Print and shaded views of the part. All mm, measured from the part's lowest x, y and z. A direction names the side the tool comes from. Give positions to 0.01 mm unless a question says otherwise; leave off trailing zeros. Loops run counter-clockwise (first coordinate to the right, second up) from the corner with the lowest first, then second, coordinate; pieces in that order, holes last. Notation, with made-up numbers: (56.5, 18) - (88.5, 18) arc R36 ccw to (88.5, 55) - close; hole circle Ø10 at (46.5, 87). An arc over 180 degrees is marked (long way). Return JSON: item names as keys, results as strings.
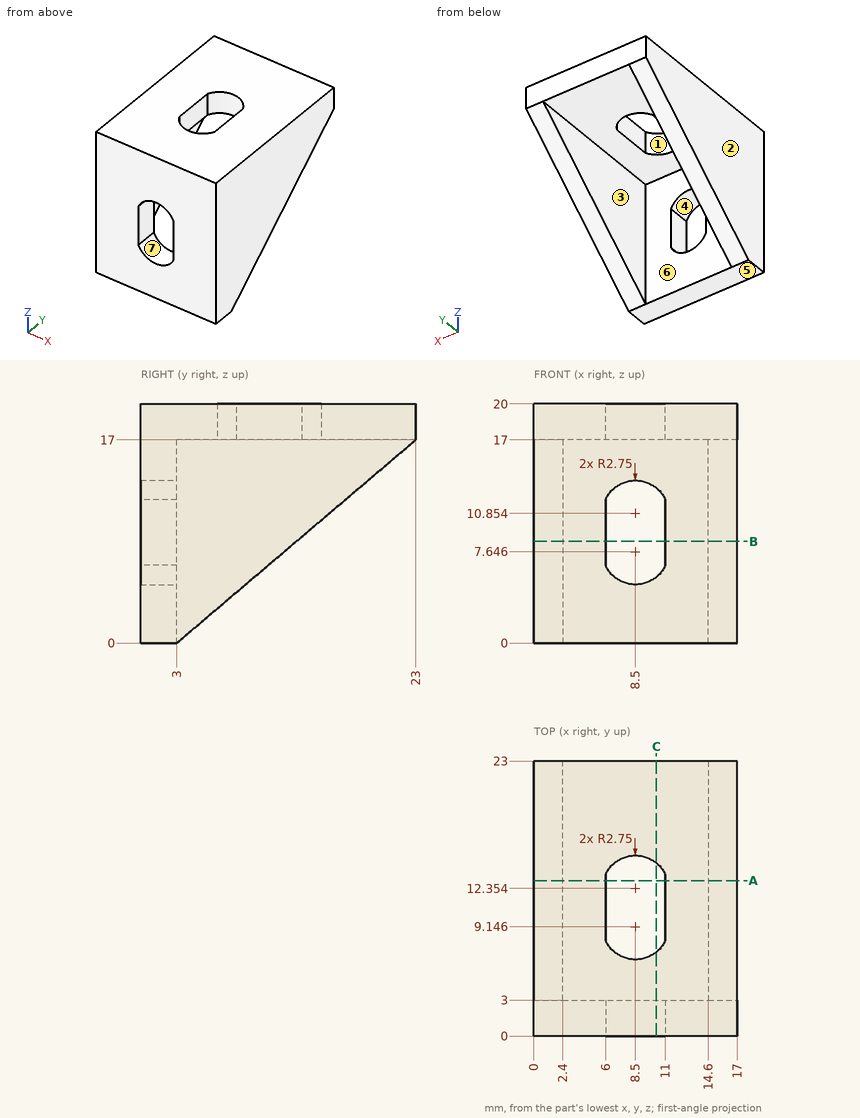
1. Pull direction Z, two halves, no side cores. Call the marked faces 4, 5, 6 and 7: +Z half, -Z half, draft (parallel to the pull), parting line (faces both ways), or undercut.
Values follow:
{"face 4": "undercut", "face 5": "-Z half", "face 6": "draft", "face 7": "undercut"}
2. Which spindle directions (+Z, -Z, +X, -X, +Y, -Y) get a long thin tool onto all of the face, cutting with end or side? Do the marked faces 1, 2 and 3. Say none if no direction does.
Values follow:
{"face 1": "+Z, -Z", "face 2": "+Z, -Z, -X, +Y, -Y", "face 3": "-Z, +Y"}
3. Cut at B-B, the plane z = 8.5. Write the cut outline in (x, y).
Values follow:
{"outline": "(0, 0) - (6, 0) - (6, 3) - (2.4, 3) - (2.4, 13) - (0, 13) - close; (11, 0) - (17, 0) - (17, 13) - (14.6, 13) - (14.6, 3) - (11, 3) - close"}
4. Drill centre lines: probe 1 along X at (y, z) = (12.5, 13.75); probe 2 along Z at (x, y) = (14.25, 21.75); probe 3 along Y at (x, z) = (8, 15.75). Where is each one in solid material? Low to high.
Values follow:
{"probe 1": "x = 0 to 2.4, 14.6 to 17", "probe 2": "z = 17 to 20", "probe 3": "y = 0 to 3"}
5. Cut at A-A, the plane y = 13. Write the cut outline in (x, z).
Values follow:
{"outline": "(0, 8.5) - (2.4, 8.5) - (2.4, 17) - (6, 17) - (6, 20) - (0, 20) - close; (11, 17) - (14.6, 17) - (14.6, 8.5) - (17, 8.5) - (17, 20) - (11, 20) - close"}
6. Cut at C-C, the plane x = 10.25. Write the cut outline in (y, z) (1 decimal).
Values follow:
{"outline": "(0, 0) - (3, 0) - (3, 5.5) - (0, 5.5) - close; (0, 13) - (3, 13) - (3, 17) - (7, 17) - (7, 20) - (0, 20) - close; (14.5, 17) - (23, 17) - (23, 20) - (14.5, 20) - close"}
7. Drop a flat-ended pin along its axis: P1, Ø1, axis at x = 7.5, y = 15, coming from the -Z side. Give the stop position or say it passes through.
Values follow:
{"P1": "stops at z = 17"}
